```python
from build123d import *

# Parameters (mm, degrees)
SKETCH_1_W          = 4
SKETCH_1_H          = 21
SKETCH_1_H_2        = 8
EXTRUDE_1_DEPTH     = 4
SKETCH_1_7_W        = 44.5
SKETCH_1_7_H        = 8
EXTRUDE_2_DEPTH     = 3.5
SKETCH_2_W          = 18.5
SKETCH_2_H          = 1.5
CUT_EXTRUDE_1_DEPTH = 37.7704025
SKETCH_2_3_W        = 2.5
SKETCH_2_3_H        = 1.5
EXTRUDE_4_DEPTH     = 29
FILLET_1_R          = 1
FILLET_2_R          = 1.5
FILLET_3_R          = 1
REVOLVE_2_ANGLE     = 17
CUT_EXTRUDE_5_DEPTH = 70.125096927
REVOLVE_1_ANGLE     = 2


with BuildPart() as part:
    # Sketch 1 → Extrude 1 (new body)
    with BuildSketch(Plane(origin=(0, 0, 0), x_dir=(1, 0, 0), z_dir=(0, 1, 0))):
        with Locations((-15.75, -4)):
            Rectangle(SKETCH_1_W, SKETCH_1_H)
        with Locations((15.75, -4)):
            Rectangle(SKETCH_1_W, SKETCH_1_H)
        with Locations((15.75, 10.5)):
            Rectangle(SKETCH_1_W, SKETCH_1_H_2)
        with Locations((-15.75, 10.5)):
            Rectangle(SKETCH_1_W, SKETCH_1_H_2)
    extrude(amount=EXTRUDE_1_DEPTH)

    # Sketch 1_7 → Extrude 2 (add)
    with BuildSketch(Plane(origin=(0, 0, 0), x_dir=(1, 0, 0), z_dir=(0, 1, 0))):
        with Locations((0, 10.5)):
            Rectangle(SKETCH_1_7_W, SKETCH_1_7_H)
    extrude(amount=EXTRUDE_2_DEPTH)

    # Sketch 2 → Cut-Extrude 1 (cut, through all)
    with BuildSketch(Plane(origin=(0, 0, -14.5), x_dir=(-1, 0, 0), z_dir=(0, 0, -1))):
        with Locations((0, 2.75)):
            Rectangle(SKETCH_2_W, SKETCH_2_H)
        Polygon((13.25, 3.5), (9.25, 3.5), (9.25, 2), align=None)
        Polygon((-9.25, 3.5), (-13.25, 3.5), (-9.25, 2), align=None)
        Polygon((-22.25, 3.5), (-22.25, 2), (-18.25, 3.5), align=None)
        Polygon((22.25, 3.5), (18.25, 3.5), (22.25, 2), align=None)
    extrude(amount=-CUT_EXTRUDE_1_DEPTH, mode=Mode.SUBTRACT)

    # Sketch 2_3 → Extrude 4 (add, through all)
    with BuildSketch(Plane(origin=(0, 0, -14.5), x_dir=(-1, 0, 0), z_dir=(0, 0, -1))):
        with Locations((-15.75, 7.25)):
            Rectangle(SKETCH_2_3_W, SKETCH_2_3_H)
        Polygon((-15, 6.5), (-16.5, 6.5), (-16.5, 4), (-15.75, 4), (-15, 4), align=None)
        with Locations((15.75, 7.25)):
            Rectangle(SKETCH_2_3_W, SKETCH_2_3_H)
        Polygon((16.5, 6.5), (15, 6.5), (15, 4), (15.75, 4), (16.5, 4), align=None)
    extrude(amount=-EXTRUDE_4_DEPTH)

    # Fillet 1
    # the kernel refuses this fillet: 1 mm, written as the material it adds along each edge
    with BuildSketch(Plane(origin=(-16.5, 6.5, -14.5), x_dir=(-1, 0, 0), z_dir=(0, 0, 1)), Plane(origin=(15, 6.5, -14.5), x_dir=(-1, 0, 0), z_dir=(0, 0, 1))) as fillet_1_piece_1:
        with BuildLine():
            CenterArc((1, 0.866025404), FILLET_1_R, 180, 60)
            Line((0, 0.866025404), (-0.02, 0.866025404))
            Line((-0.02, 0.866025404), (-0.02, 0))
            Line((-0.02, 0), (0, -0.02))
            ThreePointArc((0, -0.02), (0.25, -0.02), (0.49, -0.017320508))
            Line((0.49, -0.017320508), (0.5, 0))
        make_face()
    extrude(amount=29)
    with BuildSketch(Plane(origin=(-15, 6.5, -14.5), x_dir=(0, -1, 0), z_dir=(0, 0, 1)), Plane(origin=(16.5, 6.5, -14.5), x_dir=(0, -1, 0), z_dir=(0, 0, 1))) as fillet_1_piece_2:
        with BuildLine():
            CenterArc((0.866025404, 1), FILLET_1_R, 210, 60)
            Line((0, 0.5), (-0.017320508, 0.49))
            ThreePointArc((-0.017320508, 0.49), (-0.02, 0.25), (-0.02, 0))
            Line((-0.02, 0), (0, -0.02))
            Line((0, -0.02), (0.866025404, -0.02))
            Line((0.866025404, -0.02), (0.866025404, 0))
        make_face()
    extrude(amount=29)

    # Fillet 2
    # the kernel refuses this fillet: 1.5 mm, written as the material it adds along each edge
    with BuildSketch(Plane(origin=(16.5, 4, -14.5), x_dir=(1, 0, 0), z_dir=(0, 0, 1))) as fillet_2_piece_1:
        with BuildLine():
            CenterArc((1.5, 1.479019946), FILLET_2_R, 180, 80.405931773)
            Line((0, 1.479019946), (-0.03, 1.479019946))
            Line((-0.03, 1.479019946), (-0.03, 0))
            Line((-0.03, 0), (0, -0.03))
            ThreePointArc((0, -0.03), (0.625, -0.03), (1.245, -0.029580399))
            Line((1.245, -0.029580399), (1.25, 0))
        make_face()
    extrude(amount=29)
    with BuildSketch(Plane(origin=(15, 4, -14.5), x_dir=(0, 1, 0), z_dir=(0, 0, 1)), Plane(origin=(-16.5, 4, -14.5), x_dir=(0, 1, 0), z_dir=(0, 0, 1))) as fillet_2_piece_2:
        with BuildLine():
            CenterArc((1.479019946, 1.5), FILLET_2_R, 189.594068227, 80.405931773)
            Line((0, 1.25), (-0.029580399, 1.245))
            ThreePointArc((-0.029580399, 1.245), (-0.03, 0.625), (-0.03, 0))
            Line((-0.03, 0), (0, -0.03))
            Line((0, -0.03), (1.479019946, -0.03))
            Line((1.479019946, -0.03), (1.479019946, 0))
        make_face()
    extrude(amount=29)
    with BuildSketch(Plane(origin=(-15, 4, -14.5), x_dir=(0, 1, 0), z_dir=(0, 0, 1))) as fillet_2_piece_3:
        with BuildLine():
            CenterArc((1.479019946, -1.5), FILLET_2_R, 90, 80.405931773)
            Line((0, -1.25), (-0.029580399, -1.245))
            ThreePointArc((-0.029580399, -1.245), (-0.03, -0.625), (-0.03, 0))
            Line((-0.03, 0), (0, 0.03))
            Line((0, 0.03), (1.479019946, 0.03))
            Line((1.479019946, 0.03), (1.479019946, 0))
        make_face()
    extrude(amount=29)

    # Fillet 3
    fillet_3_edges = [part.edges().sort_by_distance(p)[0] for p in [
        (14.5, 8, 0),
        (17, 8, 0),
        (-17, 8, 0),
        (-14.5, 8, 0),
    ]]
    fillet(fillet_3_edges, radius=FILLET_3_R)

    # Sketch 7 → Revolve 2 (revolve)
    with BuildSketch(Plane(origin=(0, 0, -14.5), x_dir=(-1, 0, 0), z_dir=(0, 0, -1))):
        with BuildLine():
            Line((-17.75, 3.5), (-17.75, 0))
            Line((-17.75, 0), (-13.75, 0))
            Line((-13.75, 0), (-13.75, 3.5))
            Line((-13.75, 3.5), (-13.75, 4))
            ThreePointArc((-13.75, 4), (-14.645643924, 4.510774109), (-15, 5.479019946))
            Line((-15, 5.479019946), (-15, 5.633974596))
            ThreePointArc((-15, 5.633974596), (-14.866025404, 6.133974596), (-14.5, 6.5))
            Line((-14.5, 6.5), (-14.5, 7))
            ThreePointArc((-14.5, 7), (-14.792893219, 7.707106781), (-15.5, 8))
            Line((-15.5, 8), (-16, 8))
            ThreePointArc((-16, 8), (-16.707106781, 7.707106781), (-17, 7))
            Line((-17, 7), (-17, 6.5))
            ThreePointArc((-17, 6.5), (-16.633974596, 6.133974596), (-16.5, 5.633974596))
            Line((-16.5, 5.633974596), (-16.5, 5.479019946))
            ThreePointArc((-16.5, 5.479019946), (-16.854356076, 4.510774109), (-17.75, 4))
            Line((-17.75, 4), (-17.75, 3.5))
        make_face()
        with BuildLine():
            Line((13.75, 3.5), (13.75, 0))
            Line((13.75, 0), (17.75, 0))
            Line((17.75, 0), (17.75, 3.5))
            Line((17.75, 3.5), (17.75, 4))
            ThreePointArc((17.75, 4), (16.854356076, 4.510774109), (16.5, 5.479019946))
            Line((16.5, 5.479019946), (16.5, 5.633974596))
            ThreePointArc((16.5, 5.633974596), (16.633974596, 6.133974596), (17, 6.5))
            Line((17, 6.5), (17, 7))
            ThreePointArc((17, 7), (16.707106781, 7.707106781), (16, 8))
            Line((16, 8), (15.5, 8))
            ThreePointArc((15.5, 8), (14.792893219, 7.707106781), (14.5, 7))
            Line((14.5, 7), (14.5, 6.5))
            ThreePointArc((14.5, 6.5), (14.866025404, 6.133974596), (15, 5.633974596))
            Line((15, 5.633974596), (15, 5.479019946))
            ThreePointArc((15, 5.479019946), (14.645643924, 4.510774109), (13.75, 4))
            Line((13.75, 4), (13.75, 3.5))
        make_face()
    revolve(axis=Axis((-200, 10, -14.5), (0, 1, 0)), revolution_arc=REVOLVE_2_ANGLE)

    # Sketch 5_2 → Cut-Extrude 5 (cut, through all)
    with BuildSketch(Plane(origin=(0, 0, -14.5), x_dir=(-1, 0, 0), z_dir=(0, 0, -1))):
        with BuildLine():
            Line((17, 6.5), (17, 7))
            ThreePointArc((17, 7), (16.707106781, 7.707106781), (16, 8))
            Line((16, 8), (15.5, 8))
            ThreePointArc((15.5, 8), (14.792893219, 7.707106781), (14.5, 7))
            Line((14.5, 7), (14.5, 6.5))
            ThreePointArc((14.5, 6.5), (14.866025404, 6.133974596), (15, 5.633974596))
            Line((15, 5.633974596), (15, 5.479019946))
            ThreePointArc((15, 5.479019946), (14.645643924, 4.510774109), (13.75, 4))
            Line((13.75, 4), (13.75, 3.5))
            Line((13.75, 3.5), (13.25, 3.5))
            Line((13.25, 3.5), (9.25, 2))
            Line((9.25, 2), (-9.25, 2))
            Line((-9.25, 2), (-13.25, 3.5))
            Line((-13.25, 3.5), (-13.75, 3.5))
            Line((-13.75, 3.5), (-13.75, 4))
            ThreePointArc((-13.75, 4), (-14.645643924, 4.510774109), (-15, 5.479019946))
            Line((-15, 5.479019946), (-15, 5.633974596))
            ThreePointArc((-15, 5.633974596), (-14.866025404, 6.133974596), (-14.5, 6.5))
            Line((-14.5, 6.5), (-14.5, 7))
            ThreePointArc((-14.5, 7), (-14.792893219, 7.707106781), (-15.5, 8))
            Line((-15.5, 8), (-16, 8))
            ThreePointArc((-16, 8), (-16.707106781, 7.707106781), (-17, 7))
            Line((-17, 7), (-17, 6.5))
            ThreePointArc((-17, 6.5), (-16.633974596, 6.133974596), (-16.5, 5.633974596))
            Line((-16.5, 5.633974596), (-16.5, 5.479019946))
            ThreePointArc((-16.5, 5.479019946), (-16.854356076, 4.510774109), (-17.75, 4))
            Line((-17.75, 4), (-17.75, 3.5))
            Line((-17.75, 3.5), (-18.25, 3.5))
            Line((-18.25, 3.5), (-22.25, 2))
            Line((-22.25, 2), (-22.25, 0))
            Line((-22.25, 0), (22.25, 0))
            Line((22.25, 0), (22.25, 2))
            Line((22.25, 2), (18.25, 3.5))
            Line((18.25, 3.5), (17.75, 3.5))
            Line((17.75, 3.5), (17.75, 4))
            ThreePointArc((17.75, 4), (16.854356076, 4.510774109), (16.5, 5.479019946))
            Line((16.5, 5.479019946), (16.5, 5.633974596))
            ThreePointArc((16.5, 5.633974596), (16.633974596, 6.133974596), (17, 6.5))
        make_face()
    extrude(amount=-CUT_EXTRUDE_5_DEPTH, mode=Mode.SUBTRACT)


with BuildPart() as cut_extrude_5_piece_1:
    # of the separate pieces the step leaves, piece 1, a body of its own (cut_extrude_5_pieces)
    add(part.part.solids().sort_by_distance((13.75, 0, -14.5))[0])



with BuildPart() as cut_extrude_5_piece_2:
    # of the separate pieces the step leaves, piece 2, a body of its own (cut_extrude_5_pieces)
    add(part.part.solids().sort_by_distance((-13.75, 4, -14.5))[0])


with BuildPart() as cut_extrude_5_piece_1_1:
    add(cut_extrude_5_piece_1.part)

    add(cut_extrude_5_piece_2.part)  # Revolve 1 merges Cut-Extrude 5 piece 2
    # Sketch 5 → Revolve 1 (revolve)
    with BuildSketch(Plane(origin=(0, 0, -14.5), x_dir=(-1, 0, 0), z_dir=(0, 0, -1))):
        with BuildLine():
            Line((17, 6.5), (17, 7))
            ThreePointArc((17, 7), (16.707106781, 7.707106781), (16, 8))
            Line((16, 8), (15.5, 8))
            ThreePointArc((15.5, 8), (14.792893219, 7.707106781), (14.5, 7))
            Line((14.5, 7), (14.5, 6.5))
            ThreePointArc((14.5, 6.5), (14.866025404, 6.133974596), (15, 5.633974596))
            Line((15, 5.633974596), (15, 5.479019946))
            ThreePointArc((15, 5.479019946), (14.645643924, 4.510774109), (13.75, 4))
            Line((13.75, 4), (13.75, 3.5))
            Line((13.75, 3.5), (13.25, 3.5))
            Line((13.25, 3.5), (9.25, 2))
            Line((9.25, 2), (-9.25, 2))
            Line((-9.25, 2), (-13.25, 3.5))
            Line((-13.25, 3.5), (-13.75, 3.5))
            Line((-13.75, 3.5), (-13.75, 4))
            ThreePointArc((-13.75, 4), (-14.645643924, 4.510774109), (-15, 5.479019946))
            Line((-15, 5.479019946), (-15, 5.633974596))
            ThreePointArc((-15, 5.633974596), (-14.866025404, 6.133974596), (-14.5, 6.5))
            Line((-14.5, 6.5), (-14.5, 7))
            ThreePointArc((-14.5, 7), (-14.792893219, 7.707106781), (-15.5, 8))
            Line((-15.5, 8), (-16, 8))
            ThreePointArc((-16, 8), (-16.707106781, 7.707106781), (-17, 7))
            Line((-17, 7), (-17, 6.5))
            ThreePointArc((-17, 6.5), (-16.633974596, 6.133974596), (-16.5, 5.633974596))
            Line((-16.5, 5.633974596), (-16.5, 5.479019946))
            ThreePointArc((-16.5, 5.479019946), (-16.854356076, 4.510774109), (-17.75, 4))
            Line((-17.75, 4), (-17.75, 3.5))
            Line((-17.75, 3.5), (-18.25, 3.5))
            Line((-18.25, 3.5), (-22.25, 2))
            Line((-22.25, 2), (-22.25, 0))
            Line((-22.25, 0), (22.25, 0))
            Line((22.25, 0), (22.25, 2))
            Line((22.25, 2), (18.25, 3.5))
            Line((18.25, 3.5), (17.75, 3.5))
            Line((17.75, 3.5), (17.75, 4))
            ThreePointArc((17.75, 4), (16.854356076, 4.510774109), (16.5, 5.479019946))
            Line((16.5, 5.479019946), (16.5, 5.633974596))
            ThreePointArc((16.5, 5.633974596), (16.633974596, 6.133974596), (17, 6.5))
        make_face()
    revolve(axis=Axis((-200, 10, -14.5), (0, 1, 0)), revolution_arc=REVOLVE_1_ANGLE)


solid = cut_extrude_5_piece_1_1.part
```
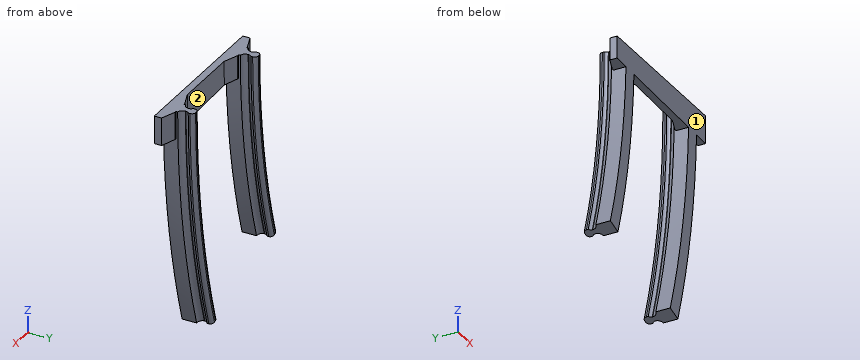
Model file for the job. Use its own axes, mm. Face numbers are marked on the shaded views. Round coordinates to 2 decimals unless told otherwise and drop trailing zeros. Write each loop counter-clockwise with the first axis right and the second up, starting at its lowest first coordinate (ties: lowest second). Pieces come first, ordered by that corner, then holes. Notation, with made-up numbers: M 17,59.25 L 53,59.25 A18 cw 53,69.25 Z; hole C -3,-24 d10. An arc over 180 degrees is marked long. Put each result on its own line as item: value.
Item 1: Cut at C-C (x = -7). List the corners of the cut face in (y, z).
Responses:
outline: M 0,-21.24 L 2,-21.24 L 2,-14.5 L 0,-14.5 Z
Item 2: Probe L1, parallel to X at y = 1, z = -39.5; L2, parallel to X at y = 3.75, z = -55; L3, parallel to Y at x = -22, z = -67.5. List the from-to ranges inside material, lowest first. Write a range as from..to.
Responses:
L1: -19.47..-15.44, 12.28..16.31
L2: -22.31..-18.21, 9.88..13.95
L3: 0..4.2
Item 3: Flat gauge pins, fed straight in: P1, Ø6, axis at x = -14, z = -62.5, coming from the -Y side; P2, Ø6, axis at x = -4, z = -16.5, coming from the +Y side; P3, Ø1, axis at y = 5, z = -38, coming from the -X side; P4, Ø0.7, axis at x = -18, z = -17.5, coming from the +Y side. Where does each tip first touch, or does it go through?
Responses:
P1: through
P2: y = 2
P3: x = -18.38
P4: y = 4.03
Item 4: Cut at B-B (y = 1). List the corners of the cut face in (x, z), and give its area (3 significant figures).
Responses:
outline: M -25.71,-67.78 L -21.89,-68.95 A186.25 ccw -13.86,-21 L 13.62,-21.96 A213.75 cw 4.41,-76.99 L 8.24,-78.16 A217.75 ccw 17.62,-22.1 L 22.11,-22.26 A222.25 ccw 22.25,-14.5 L -22.25,-14.5 A177.75 cw -22.36,-20.7 L -17.86,-20.86 A182.25 cw Z
area: 730 mm²
Item 5: Mould opens along X. For the marked faces 1 and 2 say: +X half, -X half, draft (parallel to the pull), parting line (faces both ways), or undercut.
Responses:
face 1: draft
face 2: undercut
Item 6: Cut at A-A (y = 4.75). List the corners of the cut face in (x, z).
Responses:
outline: M -24.7,-68.09 L -22.9,-68.64 A185.19 ccw -14.81,-14.5 L -16.69,-14.5 A183.31 cw Z; M 5.42,-77.3 L 7.22,-77.85 A216.69 ccw 16.69,-14.5 L 14.81,-14.5 A214.81 cw Z
